Part model, mm, in its own coordinate system. A direction names the side the tool comes from. Give positions to 0.01 mm unless a question says otherwise; leave off trailing zeros. Answer in a Markdown table with one row per item.
from build123d import *

# Parameters (mm, degrees)
FILLET1_R          = 6.35
CUT_EXTRUDE2_DEPTH = 5.715


with BuildPart() as part:
    # Loft1: read off the stored shape, not the designer's step
    # Loft1: loft between two sections, ruled curve by curve
    loft1_from = [
        Edge.make_bspline([(175.269753602, 13.29140622, 0), (165.836250903, 10.800407431, 0), (146.733604162, 6.768636817, 0), (117.705631888, 3.120825545, 0), (88.515569293, 1.298481639, 0), (69.014979931, 0.896470859, 0), (55.76421182, 0.761993128, 0), (48.774937515, 0.717177079, 0), (38.290373313, 0.701329652, 0), (27.805353703, 0.707699483, 0), (17.319910015, 0.713085206, 0), (6.83407663, 0.722118469, 0), (-7.147508406, 0.739950104, 0), (-24.625279721, 0.778748607, 0), (-45.599536509, 0.865679132, 0), (-66.57427479, 1.007789933, 0), (-87.548981294, 1.219546921, 0), (-115.514221109, 1.6142682, 0), (-150.466857604, 2.354791987, 0), (-192.394333089, 3.75520411, 0), (-234.292384281, 5.782786145, 0), (-262.192310795, 7.628406717, 0), (-276.130119323, 8.693130358, 0)], [0, 0, 0, 0, 0.0646771, 0.1293542, 0.1940313, 0.2587084, 0.2587084, 0.281873762, 0.305039125, 0.328204487, 0.35136985, 0.374535212, 0.397700575, 0.4440313, 0.490362025, 0.53669275, 0.583023475, 0.6293542, 0.72201565, 0.8146771, 0.90733855, 1, 1, 1, 1], 3),
        Edge.make_bspline([(-276.130119323, 8.693130358, 0), (-268.53787532, 9.576768707, 0), (-253.325399224, 11.344499336, 0), (-230.431819466, 13.984673016, 0), (-207.472747934, 16.599459007, 0), (-188.293872161, 18.747068462, 0), (-172.928345638, 20.442413166, 0), (-161.394414944, 21.702112718, 0), (-149.852162971, 22.949878112, 0), (-138.303049105, 24.185400988, 0), (-126.749160881, 25.414250719, 0), (-115.192581437, 26.642009102, 0), (-103.635319012, 27.873545783, 0), (-92.079421128, 29.114032776, 0), (-82.4523943, 30.15987089, 0), (-74.753639148, 31.007237325, 0), (-68.981311413, 31.649138297, 0), (-63.211054502, 32.298649993, 0), (-57.443210697, 32.957070927, 0), (-51.678207111, 33.626346988, 0), (-45.916440626, 34.308134914, 0), (-40.158566872, 35.006057107, 0), (-34.405025776, 35.721868628, 0), (-28.65726222, 36.464938228, 0), (-22.912163066, 37.208891257, 0), (-17.164494437, 37.912252593, 0), (-11.409460822, 38.52679641, 0), (-5.649439363, 39.060124365, 0), (0.112709129, 39.531603667, 0), (5.875152486, 39.955359252, 0), (11.636225955, 40.347755751, 0), (17.394685212, 40.723251, 0), (23.149306668, 41.097541248, 0), (28.899044879, 41.484229227, 0), (34.642434767, 41.900999198, 0), (40.378877605, 42.351270671, 0), (46.114635135, 42.749637865, 0), (51.851500917, 43.055266027, 0), (59.500067158, 43.326067455, 0), (69.055892317, 43.378352696, 0), (80.491984345, 42.872950191, 0), (88.069711352, 42.111461167, 0), (96.99345827, 41.022920564, 0), (106.798051302, 39.527027067, 0), (120.757492461, 36.908252937, 0), (134.380844207, 33.958325891, 0), (143.515206323, 31.743252941, 0), (149.29638768, 29.715848138, 0), (151.784819047, 28.759100363, 0), (156.573051684, 26.578927821, 0), (162.27208079, 23.407349715, 0), (168.873329947, 18.939330848, 0), (173.160310936, 15.339346478, 0), (175.269753602, 13.29140622, 0)], [0, 0, 0, 0, 0.049341751, 0.098683502, 0.148025253, 0.197367004, 0.22203788, 0.246708755, 0.271379631, 0.296050506, 0.320721382, 0.345392257, 0.370063133, 0.394734008, 0.419404884, 0.431740322, 0.444075759, 0.456411197, 0.468746635, 0.481082073, 0.49341751, 0.505752948, 0.518088386, 0.530423824, 0.542759261, 0.555094699, 0.567430137, 0.579765575, 0.592101012, 0.60443645, 0.616771888, 0.629107326, 0.641442763, 0.653778201, 0.666113639, 0.678449077, 0.690784514, 0.703119952, 0.71545539, 0.740126266, 0.764797141, 0.789468017, 0.789468017, 0.823121948, 0.856775879, 0.89042981, 0.924083742, 0.924083742, 0.933573274, 0.943062806, 0.962041871, 0.981020935, 1, 1, 1, 1], 3),
    ]
    loft1_to = [
        Edge.make_bspline([(105.998873038, 13.291406071, -171.45), (99.547178972, 11.655691815, -171.45), (86.528720121, 8.807386477, -171.45), (66.752163818, 5.81997153, -171.45), (46.823097819, 4.126992417, -171.45), (33.499454727, 3.863700867, -171.45), (24.460450661, 3.97819944, -171.45), (19.693183294, 4.042786303, -171.45), (12.542798034, 4.152256247, -171.45), (5.392928427, 4.274314749, -171.45), (-1.75642567, 4.408960717, -171.45), (-8.905264395, 4.556193059, -171.45), (-18.436362387, 4.769283228, -171.45), (-30.34894715, 5.067106419, -171.45), (-44.641989626, 5.474822285, -171.45), (-58.932973358, 5.932868481, -171.45), (-73.221898844, 6.441247299, -171.45), (-92.271055825, 7.186198942, -171.45), (-116.077358919, 8.24323151, -171.45), (-144.636691691, 9.71312147, -171.45), (-173.187791596, 11.38456436, -171.45), (-192.216363366, 12.633355108, -171.45), (-201.72927398, 13.291406071, -171.45)], [0, 0, 0, 0, 0.0646771, 0.1293542, 0.1940313, 0.2587084, 0.2587084, 0.281873762, 0.305039125, 0.328204487, 0.35136985, 0.374535212, 0.397700575, 0.4440313, 0.490362025, 0.53669275, 0.583023475, 0.6293542, 0.72201565, 0.8146771, 0.90733855, 1, 1, 1, 1], 3),
        Edge.make_bspline([(-201.72927398, 13.291406071, -171.45), (-196.706001762, 14.118734782, -171.45), (-186.669871897, 15.717039915, -171.45), (-171.640734103, 17.947797667, -171.45), (-156.630466607, 20.014212394, -171.45), (-144.132480019, 21.601236244, -171.45), (-134.13733919, 22.791040732, -171.45), (-126.641873709, 23.64360893, -171.45), (-119.146564288, 24.456514085, -171.45), (-111.650676847, 25.229878327, -171.45), (-104.153477306, 25.963823782, -171.45), (-96.654231583, 26.658472577, -171.45), (-89.152205599, 27.313946841, -171.45), (-81.646665274, 27.9303687, -171.45), (-75.388507985, 28.411611685, -171.45), (-70.379479761, 28.777128777, -171.45), (-66.621362852, 29.041524908, -171.45), (-62.861805656, 29.296176313, -171.45), (-59.100713628, 29.541079951, -171.45), (-55.337992223, 29.776232783, -171.45), (-51.573546895, 30.001631769, -171.45), (-47.8072831, 30.217273872, -171.45), (-44.039106291, 30.42315605, -171.45), (-40.268921924, 30.619275264, -171.45), (-36.496635452, 30.805628475, -171.45), (-32.722152332, 30.982212644, -171.45), (-28.945378018, 31.149024731, -171.45), (-25.166217963, 31.306061697, -171.45), (-21.384577624, 31.453320502, -171.45), (-17.600362454, 31.590798107, -171.45), (-13.813466378, 31.718470556, -171.45), (-10.023783319, 31.836313894, -171.45), (-6.231207201, 31.944304163, -171.45), (-2.435631947, 32.042417409, -171.45), (1.363048518, 32.130629675, -171.45), (5.164940272, 32.208917006, -171.45), (8.970149389, 32.277255445, -171.45), (12.778781947, 32.335621037, -171.45), (17.861664714, 32.400112757, -171.45), (24.224357154, 32.455675508, -171.45), (31.874979066, 32.482076127, -171.45), (36.986220068, 32.472698987, -171.45), (43.034735977, 32.445594637, -171.45), (50.252197512, 32.186193716, -171.45), (61.575304209, 30.990235835, -171.45), (73.03796941, 28.932962432, -171.45), (80.486980807, 27.023727732, -171.45), (85.121527508, 25.659816178, -171.45), (87.166401389, 24.993278477, -171.45), (91.228193462, 23.397991092, -171.45), (96.154779045, 20.919674072, -171.45), (101.516443745, 17.32147055, -171.45), (104.593880705, 14.655434782, -171.45), (105.998873038, 13.291406071, -171.45)], [0, 0, 0, 0, 0.049341751, 0.098683502, 0.148025253, 0.197367004, 0.22203788, 0.246708755, 0.271379631, 0.296050506, 0.320721382, 0.345392257, 0.370063133, 0.394734008, 0.419404884, 0.431740322, 0.444075759, 0.456411197, 0.468746635, 0.481082073, 0.49341751, 0.505752948, 0.518088386, 0.530423824, 0.542759261, 0.555094699, 0.567430137, 0.579765575, 0.592101012, 0.60443645, 0.616771888, 0.629107326, 0.641442763, 0.653778201, 0.666113639, 0.678449077, 0.690784514, 0.703119952, 0.71545539, 0.740126266, 0.764797141, 0.789468017, 0.789468017, 0.823121948, 0.856775879, 0.89042981, 0.924083742, 0.924083742, 0.933573274, 0.943062806, 0.962041871, 0.981020935, 1, 1, 1, 1], 3),
    ]
    loft1 = Solid(Shell([*[Face.make_surface_from_curves(loft1_from[k], loft1_to[k]) for k in range(2)], Face(Wire(loft1_from)), Face(Wire(loft1_to))]))
    add(loft1)

    # Fillet1
    fillet1_edges = [part.edges().sort_by_distance(p)[0] for p in [
        (140.63431332, 13.291406146, -85.725),
    ]]
    fillet(fillet1_edges, radius=FILLET1_R)

    # Sketch9 → Cut-Extrude2 (cut, symmetric)
    with BuildSketch(Plane(origin=(0, 19.812, 0), x_dir=(1, 0, 0), z_dir=(0, 1, 0))):
        Polygon((-7.80027398, 171.45), (-76.28723014, 171.45), (-7.016933721, 0), (61.470022439, 0), align=None)
    extrude(amount=CUT_EXTRUDE2_DEPTH, both=True, mode=Mode.SUBTRACT)


solid = part.part
(1) Pin check, flat tips, straight feed: pin 1 Ø2 at (x, z) = (-218.5, -90.5) entering from -Y; pin 2 Ø2 at (y, z) = (17.5, -115.5) entering from +X; pin 3 Ø2 at (y, z) = (18, -34) entering from +X; pin 4 Ø8 at (x, y) = (-11, 21.5) entering from +Z. Stop position of each tip, or through.
Recorded:
| item | result |
|---|---|
| pin 1 | stops at y = 9.76 |
| pin 2 | stops at x = 120.98 |
| pin 3 | stops at x = 154.2 |
| pin 4 | stops at z = 0 |
(2) Drill centre lines: line 1 along Y through (x, z) = (57.5, -9); line 2 along Y through (x, z) = (-11, -91); line 3 along Y through (x, z) = (-92.5, -102.5). Where is each one in solid material? Low to high.
Recorded:
| item | result |
|---|---|
| line 1 | y = 0.96 to 14.1, 25.53 to 42.71 |
| line 2 | y = 2.86 to 14.1, 25.53 to 35.26 |
| line 3 | y = 4.71 to 27.77 |
(3) Which spindle directions (+Z, -Z, +X, -X, +Y, -Y) get a long thin tool onto all of the face, cutting with end or side? Do faces 3 (the face through (-17, 12, -171.45)), 4 (the face through (-8, 25.527, -87)). Say none if no direction does.
Recorded:
| item | result |
|---|---|
| face 3 | -Z, +X, -X, +Y, -Y |
| face 4 | none |
(4) Pull direction X, two halves, no side cores. Call faces 1 (the face through (27.32, 19.89, -84.52)), 2 (the face through (-2, 13, 0)): +X half, -X half, draft (parallel to the pull), parting line (faces both ways), or undercut.
Recorded:
| item | result |
|---|---|
| face 1 | undercut |
| face 2 | draft |
